Part model, mm, in its own coordinate system. Round coordinates to 2 decimals unless told otherwise and drop trailing zeros. Write each loop counter-clockwise with the first axis right and the second up, starting at its lowest first coordinate (ties: lowest second). Pieces come first, ordered by that corner, then holes. Notation, with made-up numbers: (-22.5, 87) -> (30.5, 87) arc R18 cw to (30.5, 119) -> close; hole circle Ø9 at (70, -17). An arc over 180 degrees is marked (long way). Return JSON: item names as keys, results as strings. Group by question number.
(1) Saw through at C-C (y = 50). List the corners of the cut face in (x, z), plus the area to 3 significant figures.
(2) Saw through at B-B (x = 0). List the corners of the cut face in (y, z), plus the area to 3 significant figures.
(3) Drill centre lines: L1, parallel to X at y = 50, z = 0.5; L2, parallel to Y at x = -10, z = 1.15; L3, parallel to Y at x = 28.5, z = 1.7. Where is each one in solid material? Low to high. Write a range as from..to.
(4) Drop flat-ended pins along their axis: pin 1 Ø1.9 at (x, y) = (28.64, -11.86) entering from +Z; pin 2 Ø0.7 at (y, z) = (62, 1.5) entering from -X; pin 3 Ø0.7 at (y, z) = (63, 1.5) entering from +X. Give the stop position or say it passes through.
(5) Saw through at D-D (x = 8.5). List the corners of the cut face in (y, z).
(6) Saw through at A-A (y = 0). List the corners of the cut face in (x, z).
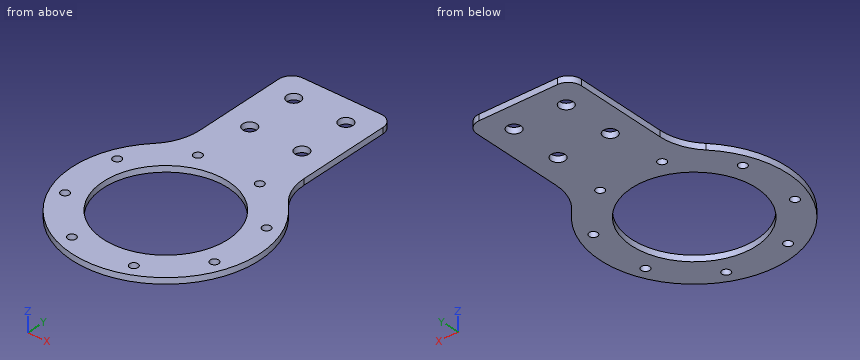
Autodesk Inventor part; units mm, degrees
ref_plane "YZ Plane" through (0, 0, 0) normal (1, 0, 0) x (0, 1, 0)
ref_plane "XZ Plane" through (0, 0, 0) normal (0, 1, 0) x (-1, 0, 0)
ref_plane "XY Plane" through (0, 0, 0) normal (0, 0, 1) x (1, 0, 0)
sketch "スケッチ1" plane through (0, 0, 0) normal (0, 0, 1) x (1, 0, 0)
  arc A0 (-20, 29.9333) -> (20, 29.9333) centre (0, 0) ccw
  line L0 (-20, -80) -> (20, -80)
  line L1 (20, -80) -> (20, 80)
  line L2 (20, 80) -> (-20, 80)
  line L3 (-20, 80) -> (-20, -80)
  line L4 (-20, -80) -> (20, 80) construction
  line L5 (20, -80) -> (-20, 80) construction
  dimension "d0" = 72
  dimension "d1" = 80
  dimension "d2" = 40
extrude "プレート1" add sketch "スケッチ1" along normal blind 2.3 contours L3 A0 | L3 L2 L1 A0 | L1 A0
sketch "スケッチ2" plane through (0, 0, 2.3) normal (0, 0, 1) x (1, 0, 0)
  circle A0 centre (0, 0) radius 31
  point P0 (-28.6403, -11.8632)
  point P1 (-11.8632, -28.6403)
  point P2 (11.8632, -28.6403)
  point P3 (28.6403, -11.8632)
  point P4 (28.6403, 11.8632)
  point P5 (11.8632, 28.6403)
  point P6 (-11.8632, 28.6403)
  point P7 (-28.6403, 11.8632)
  dimension "d5" = 62
  dimension "d8" = 360
  dimension "d34" = 0
hole "穴1" at (-28.6403, 11.8632, 2.3) at (-11.8632, 28.6403, 2.3) at (11.8632, 28.6403, 2.3) at (28.6403, 11.8632, 2.3) at (28.6403, -11.8632, 2.3) at (11.8632, -28.6403, 2.3) at (-11.8632, -28.6403, 2.3) at (-28.6403, -11.8632, 2.3) direction (0, 0, -1) diameter 3.242 end through all
sketch "スケッチ4" plane through (0, 0, 2.3) normal (0, 0, 1) x (1, 0, 0)
  line L0 (10, 50) -> (-10, 50)
  line L1 (-10, 50) -> (-10, 70)
  line L2 (-10, 70) -> (10, 70)
  line L3 (10, 70) -> (10, 50)
  line L4 (10, 50) -> (-10, 70) construction
  line L5 (-10, 50) -> (10, 70) construction
  line L6 (-20, 80) -> (20, 80)
  circle A0 centre (0, 0) radius 72.5
  point P0 (0, 60)
  point P1 (0, 60)
  dimension "d21" = 20
  dimension "d22" = 10
  dimension "d33" = 145
  dimension "d38" = 20
hole "穴2" at (-10, 70, 2.3) at (10, 70, 2.3) at (-10, 50, 2.3) at (10, 50, 2.3) direction (0, 0, -1) diameter 5.3 end through all
fillet "コーナーR2" radius 5 2 edges at (-20, 80, 1.15) (20, 80, 1.15)
sketch "スケッチ5" plane through (0, 0, 2.3) normal (0, 0, 1) x (1, 0, 0)
  circle A0 centre (0, 0) radius 24
  dimension "d35" = 48
extrude "押し出し2" cut sketch "スケッチ5" against normal blind 10
fillet "コーナーR3" radius 20 2 edges at (20, 29.9333, 1.15) (-20, 29.9333, 1.15)
equation "\"d16\" = Thickness"
equation "\"d3\" = Thickness"
equation "\"BendRadius\" = Thickness"
equation "\"BendReliefWidth\" = Thickness"
equation "\"BendReliefDepth\" = 0.5 * Thickness"
equation "\"CornerReliefSize\" = 4 * Thickness"
equation "\"MinimumRemnant\" = 2 * Thickness"
equation "\"TransitionRadius\" = BendRadius"
equation "\"JacobiRadiusSize\" = BendRadius"
equation "\"GapSize\" = Thickness"
properties part number "scara-plate9" material "鋼、炭素鋼"
Computed values:
{
 "1": {"outline": "(-20, 0) -> (-12.65, 0) -> (-12.65, 2.3) -> (-20, 2.3) -> close; (-7.35, 0) -> (7.35, 0) -> (7.35, 2.3) -> (-7.35, 2.3) -> close; (12.65, 0) -> (20, 0) -> (20, 2.3) -> (12.65, 2.3) -> close", "area": "67.6 mm2"},
 "2": {"outline": "(-36, 0) -> (-24, 0) -> (-24, 2.3) -> (-36, 2.3) -> close; (24, 0) -> (80, 0) -> (80, 2.3) -> (24, 2.3) -> close", "area": "156 mm2"},
 "3": {"L1": "-20..-12.65, -7.35..7.35, 12.65..20", "L2": "-34.58..-21.82, 21.82..47.35, 52.65..67.35, 72.65..80", "L3": "-21.99..-13.48, -10.25..10.25, 13.48..21.99"},
 "4": {"pin 1": "through", "pin 2": "x = -20", "pin 3": "x = 20"},
 "5": {"outline": "(-34.98, 0) -> (-22.44, 0) -> (-22.44, 2.3) -> (-34.98, 2.3) -> close; (22.44, 0) -> (47.82, 0) -> (47.82, 2.3) -> (22.44, 2.3) -> close; (52.18, 0) -> (67.82, 0) -> (67.82, 2.3) -> (52.18, 2.3) -> close; (72.18, 0) -> (80, 0) -> (80, 2.3) -> (72.18, 2.3) -> close"},
 "6": {"outline": "(-36, 0) -> (-24, 0) -> (-24, 2.3) -> (-36, 2.3) -> close; (24, 0) -> (36, 0) -> (36, 2.3) -> (24, 2.3) -> close"}
}
